CAD build for the part. Positions are in the model's coordinates, mm. Face numbers are marked on the shaded views. A direction names the side the tool comes from. Round coordinates to 2 decimals unless told otherwise and drop trailing zeros. Loops run counter-clockwise (first coordinate to the right, second up) from the corner with the lowest first, then second, coordinate; pieces in that order, holes last. Notation, with made-up numbers: M -15.5,35.5 L 9.5,35.5 A21 cw 9.5,63.5 Z; hole C -0.75,38 d4. An arc over 180 degrees is marked long. Use a Markdown table: item, result. Add a question column.
(1) Band-saw the part on B-B, the plane z = 0.55. Write the cut outline in (x, y), and give its area (3 significant figures).
(2) Two-plate mould, pull along X, no slides. Class the marked faces 5, 6 and 7: released by +X, released by -X, zero draft, split by the parting line, or undercut.
(3) Band-saw the part on A-A, the plane y = 1.7. Write the cut outline in (x, z), and give its area (3 significant figures).
(4) Band-saw the part on D-D, the plane y = 2.15. Write the cut outline in (x, z), and give its area (3 significant figures).
(5) Band-saw the part on C-C, the plane x = -1.25. Write the cut outline in (y, z).
(6) Flat gauge pins, fed straight in: P1, Ø1.3, axis at y = 1, z = 0.5, coming from the -X side; P2, Ø1.2, axis at x = 0.5, y = 1, coming from the -Z side; P3, Ø1.1, axis at x = 0, z = 0.5, coming from the -Y side. Where does each tip first touch, or does it go through?
(7) Which spindle directions (+Z, -Z, +X, -X, +Y, -Y) get a long thin tool onto all of the face, cutting with end or side? Do the marked faces 1, 2, 3 and 4. Say none if no direction does.
(8) Wall check: L1, parallel to X at y = -0.45, z = -1.7; L2, parallel to X at y = 1.6, z = 1.3; L3, parallel to Z at x = 1, y = 0.85. Give the ranges that are in metal, low to high.
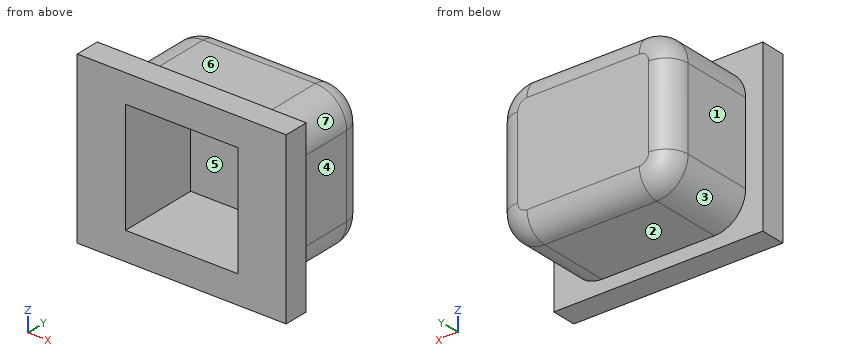
from build123d import *

# Parameters (mm, degrees)
EXTRUDE_335_DEPTH     = 3
SKETCH_2_W            = 6.7
SKETCH_2_H            = 5.4
EXTRUDE_569_DEPTH     = 0.8
SKETCH_3_W            = 3.6
SKETCH_3_H            = 3.6
CUT_EXTRUDE_834_DEPTH = 2.6
FILLET_1_R            = 0.7


with BuildPart() as part:
    # 草图1 → Extrude 335 (new body)
    with BuildSketch(Plane(origin=(0, 0, 0), x_dir=(1, 0, 0), z_dir=(0, 1, 0))):
        with BuildLine():
            Line((-1.8, -2.3), (1.8, -2.3))
            ThreePointArc((1.8, -2.3), (2.507106781, -2.007106781), (2.8, -1.3))
            Line((2.8, -1.3), (2.8, 1.3))
            ThreePointArc((2.8, 1.3), (2.507106781, 2.007106781), (1.8, 2.3))
            Line((1.8, 2.3), (-1.8, 2.3))
            ThreePointArc((-1.8, 2.3), (-2.507106781, 2.007106781), (-2.8, 1.3))
            Line((-2.8, 1.3), (-2.8, -1.3))
            ThreePointArc((-2.8, -1.3), (-2.507106781, -2.007106781), (-1.8, -2.3))
        make_face()
    extrude(amount=EXTRUDE_335_DEPTH)

    # 草图2 → Extrude 569 (add)
    with BuildSketch(Plane.XZ):
        Rectangle(SKETCH_2_W, SKETCH_2_H)
    extrude(amount=EXTRUDE_569_DEPTH)

    # 草图3 → Cut-Extrude 834 (cut)
    with BuildSketch(Plane.XZ.offset(0.8)):
        Rectangle(SKETCH_3_W, SKETCH_3_H)
    extrude(amount=-CUT_EXTRUDE_834_DEPTH, mode=Mode.SUBTRACT)

    # 圆角1
    fillet_1_edges = [part.edges().sort_by_distance(p)[0] for p in [
        (2.507106781, 3, -2.007106781),
        (0, 3, -2.3),
        (-2.507106781, 3, -2.007106781),
        (-2.8, 3, 0),
        (-2.507106781, 3, 2.007106781),
        (0, 3, 2.3),
        (2.507106781, 3, 2.007106781),
        (2.8, 3, 0),
    ]]
    fillet(fillet_1_edges, radius=FILLET_1_R)


solid = part.part
Return value:
| question | item | result |
|---|---|---|
| 1 | outline | M -3.35,-0.8 L -1.8,-0.8 L -1.8,1.8 L 1.8,1.8 L 1.8,-0.8 L 3.35,-0.8 L 3.35,0 L 2.8,0 L 2.8,2.3 A0.7 ccw 2.1,3 L -2.1,3 A0.7 ccw -2.8,2.3 L -2.8,0 L -3.35,0 Z |
| 1 | area | 12.6 mm^2 |
| 2 | face 5 | undercut |
| 2 | face 6 | zero draft |
| 2 | face 7 | released by +X |
| 3 | outline | M -2.8,-1.3 A1 ccw -1.8,-2.3 L 1.8,-2.3 A1 ccw 2.8,-1.3 L 2.8,1.3 A1 ccw 1.8,2.3 L -1.8,2.3 A1 ccw -2.8,1.3 Z; hole M -1.8,-1.8 L 1.8,-1.8 L 1.8,1.8 L -1.8,1.8 Z |
| 3 | area | 11.9 mm^2 |
| 4 | outline | M -2.8,-1.3 A1 ccw -1.8,-2.3 L 1.8,-2.3 A1 ccw 2.8,-1.3 L 2.8,1.3 A1 ccw 1.8,2.3 L -1.8,2.3 A1 ccw -2.8,1.3 Z |
| 4 | area | 24.9 mm^2 |
| 5 | outline | M -0.8,-2.7 L 0,-2.7 L 0,-2.3 L 2.3,-2.3 A0.7 ccw 3,-1.6 L 3,1.6 A0.7 ccw 2.3,2.3 L 0,2.3 L 0,2.7 L -0.8,2.7 L -0.8,1.8 L 1.8,1.8 L 1.8,-1.8 L -0.8,-1.8 Z |
| 6 | P1 | x = -2.8 |
| 6 | P2 | z = -2.3 |
| 6 | P3 | y = 1.8 |
| 7 | face 1 | +Z, -Z, -X, +Y |
| 7 | face 2 | -Z, +X, -X, +Y |
| 7 | face 3 | -Z, -X, +Y |
| 7 | face 4 | +Z, -Z, +X, +Y |
| 8 | L1 | -3.35 to -1.8, 1.8 to 3.35 |
| 8 | L2 | -2.8 to -1.8, 1.8 to 2.8 |
| 8 | L3 | -2.3 to -1.8, 1.8 to 2.3 |
